The drawing under review shows one solid part. Ordinate dimensions are in mm from its lowest x, y, z. Coordinates: 2 decimals unless noted, no trailing zeros. Write each loop counter-clockwise with the first axis right and the second up, starting at its lowest first coordinate (ties: lowest second). Pieces come first, ordered by that corner, then holes.
Q1. Add section B-B, the plane x = 28.5. Give the boundary of the cut face in (y, z).
Q2. To check wall thickness, follow probe 1 along Z at (x, y) = (13.5, 4); probe 2 along Z at (x, y) = (23, 1.75); probe 3 along X at (y, z) = (4, 114.5). State the ranges of each line that lie inside material, in increasing order.
Q3. Clearance check with flat-ended pins moving along their axes: pin 1 Ø5 at (x, y) = (4.5, 2.5) entering from +Z; pin 2 Ø2.5 at (x, y) = (11.5, 4) entering from +Z. State where each tip first meets the part, or that it passes through.
Q4. Add section A-A, the plane y = 1.75. Give the boundary of the cut face in (x, z).
Q5. Add section C-C, the plane x = 3. Give the boundary of the cut face in (y, z).
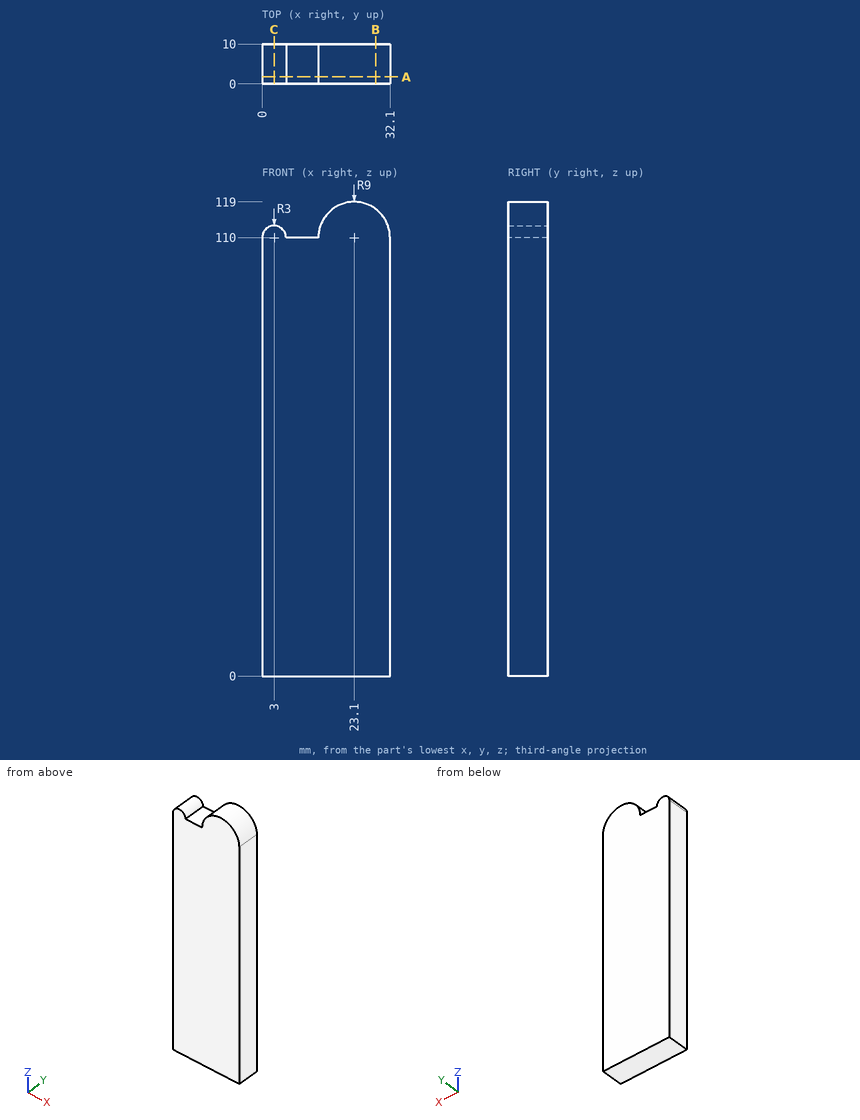
Here are the results:
1. outline: (0, 0) - (10, 0) - (10, 117.2) - (0, 117.2) - close
2. probe 1: z = 0 to 110
2. probe 2: z = 0 to 119
2. probe 3: x = 15.31 to 30.89
3. pin 1: stops at z = 113
3. pin 2: stops at z = 110
4. outline: (0, 0) - (32.1, 0) - (32.1, 110) arc R9 ccw to (14.1, 110) - (6, 110) arc R3 ccw to (0, 110) - close
5. outline: (0, 0) - (10, 0) - (10, 113) - (0, 113) - close
